Here's how the part is built. I have some questions about the finished solid (model axes, mm). A direction names the side the tool comes from. Coordinates: 2 decimals unless noted, no trailing zeros. Write each loop counter-clockwise with the first axis right and the second up, starting at its lowest first coordinate (ties: lowest second). Pieces come first, ordered by that corner, then holes. Notation, with made-up numbers: (71, -12.75) -> (84, -12.75) arc R19 ccw to (84, 13.25) -> close; hole circle Ø10 at (41.5, -22.75). An arc over 180 degrees is marked (long way). Put each result on its own line as item: value. Start each with the question number.
Item 1: If we mould it in two halves opening along X, with no side actions, what happens to faces 4 (the face through (-7.559, 62.611, 5.796)), 5 (the face through (-2.486, 65.83, 2.28)), 6 (the face through (-5, 133.35, -5))? For each: released by +X, released by -X, zero draft, split by the parting line, or undercut.
Item 2: I want a section at B-B, the plane x = 0. List the corners of the cut face in (y, z) for me (3 decimals), then the cut area to 3 significant figures.
Item 3: I want a section at C-C, the plane y = 69. List the corners of the cut face in (x, z) for me (3 decimals), then the cut area to 3 significant figures.
Item 4: I want a section at D-D, the plane x = 12. List the corners of the cut face in (y, z) for me.
Item 5: I need wall thicknesses on line 1 (Z direction, x = 0, y = 129); line 2 (Z direction, x = 0, y = 4.25) (3 decimals). Which ranges of each line are inside material? Lowest first, please. Write a range as [from, to].
Item 6: For pin 1 (10 mm diameter, centred on x = -14, z = 6.5, fed in from -Y); pin 2 (2 mm diameter, centred on x = -9, y = 14.5, fed in from +Z); pin 3 (4 mm diameter, centred on y = 113, z = 0, fed in from +X) (3 decimals), each with a flat end and sliding along its axis, tell me the tip position at first contact or that it passes through.
Item 7: I want a section at A-A, the plane z = 0. List the corners of the cut face in (x, y) for me (3 decimals), then the cut area to 3 significant figures.
Item 8: On a 3-axis mill with a long thin cutter (end or side, diameter ignored), from which of +Z, -Z, +X, -X, +Y, -Y can I reach the whole of each face in a straight line? I mean faces 1 (the face through (3, 127, 3)), 2 (the face through (3, 6.35, -3)), 3 (the face through (2, 0, 6.2)). Say none if no direction works.
from build123d import *

# Parameters (mm, degrees)
SKETCH1_R           = 9.525
BOSS_EXTRUDE1_DEPTH = 127
SKETCH2_R           = 19.05
BOSS_EXTRUDE2_DEPTH = 6.35
SKETCH3_R           = 6.35
CUT_EXTRUDE1_DEPTH  = 6.35
SKETCH4_R           = 6.35
CUT_EXTRUDE2_DEPTH  = 6.35
SKETCH5_R           = 3.3734375
CUT_EXTRUDE3_DEPTH  = 128


with BuildPart() as part:
    # Sketch1 → Boss-Extrude1 (new body)
    with BuildSketch(Plane(origin=(0, 0, 0), x_dir=(1, 0, 0), z_dir=(0, 1, 0))):
        Circle(SKETCH1_R)
    extrude(amount=BOSS_EXTRUDE1_DEPTH)

    # Sketch2 → Boss-Extrude2 (add)
    with BuildSketch(Plane(origin=(0, 127, 0), x_dir=(1, 0, 0), z_dir=(0, 1, 0))):
        Circle(SKETCH2_R)
    extrude(amount=BOSS_EXTRUDE2_DEPTH)

    # Sketch3 → Cut-Extrude1 (cut)
    with BuildSketch(Plane(origin=(0, 133.35, 0), x_dir=(1, 0, 0), z_dir=(0, 1, 0))):
        Circle(SKETCH3_R)
    extrude(amount=-CUT_EXTRUDE1_DEPTH, mode=Mode.SUBTRACT)

    # Sketch4 → Cut-Extrude2 (cut)
    with BuildSketch(Plane.XZ):
        Circle(SKETCH4_R)
    extrude(amount=-CUT_EXTRUDE2_DEPTH, mode=Mode.SUBTRACT)

    # Sketch5 → Cut-Extrude3 (cut, through all)
    with BuildSketch(Plane.XZ.offset(-6.35)):
        Circle(SKETCH5_R)
    extrude(amount=-CUT_EXTRUDE3_DEPTH, mode=Mode.SUBTRACT)


solid = part.part
Calculated:
1. face 4: split by the parting line
1. face 5: undercut
1. face 6: zero draft
2. outline: (0, -9.525) -> (127, -9.525) -> (127, -19.05) -> (133.35, -19.05) -> (133.35, -6.35) -> (127, -6.35) -> (127, -3.373) -> (6.35, -3.373) -> (6.35, -6.35) -> (0, -6.35) -> close; (0, 6.35) -> (6.35, 6.35) -> (6.35, 3.373) -> (127, 3.373) -> (127, 6.35) -> (133.35, 6.35) -> (133.35, 19.05) -> (127, 19.05) -> (127, 9.525) -> (0, 9.525) -> close
2. area: 1,690 mm2
3. outline: circle Ø19.05 at (0, 0); hole circle Ø6.747 at (0, 0)
3. area: 249 mm2
4. outline: (127, -14.8) -> (133.35, -14.8) -> (133.35, 14.8) -> (127, 14.8) -> close
5. line 1: z = [-19.05, -6.35], [6.35, 19.05]
5. line 2: z = [-9.525, -6.35], [6.35, 9.525]
6. pin 1: stops at y = 127
6. pin 2: stops at z = 5.17
6. pin 3: stops at x = 9.525
7. outline: (-19.05, 127) -> (-9.525, 127) -> (-9.525, 0) -> (-6.35, 0) -> (-6.35, 6.35) -> (-3.373, 6.35) -> (-3.373, 127) -> (-6.35, 127) -> (-6.35, 133.35) -> (-19.05, 133.35) -> close; (3.373, 6.35) -> (6.35, 6.35) -> (6.35, 0) -> (9.525, 0) -> (9.525, 127) -> (19.05, 127) -> (19.05, 133.35) -> (6.35, 133.35) -> (6.35, 127) -> (3.373, 127) -> close
7. area: 1,690 mm2
8. face 1: +Y
8. face 2: -Y
8. face 3: +Z, -Z, +X, -X, -Y
